Here's how the part is built. I have some questions about the finished solid (model axes, mm). Round coordinates to 2 decimals unless told otherwise and drop trailing zeros. Order: outer loops, then holes, each group sorted by start corner. A loop starts at its lowest first (then second) coordinate and runs counter-clockwise, first axis right, second up. Notation, with made-up numbers: (33, 86.5) -> (69, 86.5) arc R19 cw to (69, 94.5) -> close; hole circle Ø3 at (-19, -23.75). An arc over 180 degrees is marked (long way). Use a Markdown table: item, result. Add a question column.
(1) I want a section at A-A, the plane y = 4. Please give me the cut outline in (x, z), then the cut area to 3 significant figures.
(2) If I drill on probe 1 along Z at (x, y) = (-24.5, 3.75); probe 2 along Z at (x, y) = (9.5, 6); probe 3 along Y at (x, z) = (-14.5, 34.5), over which ranges is the centre line in solid material (lowest first)?
(3) I want a section at B-B, the plane x = 15. Please give me the cut outline in (y, z), then the cut area to 3 significant figures.
(4) I'm going to push a flat-ended pin straight in: P1, Ø2, axis at x = 0.5, z = 37.5, coming from the +Y side. Where does the tip first touch, or does it pass through?
from build123d import *

# Parameters (mm, degrees)
SKETCH1_W           = 80.5
SKETCH1_H           = 80
BOSS_EXTRUDE1_DEPTH = 10
CUT_EXTRUDE1_START  = -10
SKETCH2_W           = 11
SKETCH2_H           = 5
CUT_EXTRUDE1_DEPTH  = 60
CUT_EXTRUDE2_START  = -10
SKETCH3_W           = 2
SKETCH3_H           = 2
CUT_EXTRUDE2_DEPTH  = 60


with BuildPart() as part:
    # Sketch1 → Boss-Extrude1 (new body)
    with BuildSketch(Plane(origin=(0, 0, 0), x_dir=(1, 0, 0), z_dir=(0, 1, 0))):
        Rectangle(SKETCH1_W, SKETCH1_H)
    extrude(amount=BOSS_EXTRUDE1_DEPTH)

    # Sketch2 → Cut-Extrude1 (cut)
    with BuildSketch(Plane.ZY.offset(40.25).offset(CUT_EXTRUDE1_START)):
        with Locations((34.5, 7.5)):
            Rectangle(SKETCH2_W, SKETCH2_H)
    extrude(amount=-CUT_EXTRUDE1_DEPTH, mode=Mode.SUBTRACT)

    # Sketch3 → Cut-Extrude2 (cut)
    with BuildSketch(Plane.ZY.offset(40.25).offset(CUT_EXTRUDE2_START)):
        with Locations((37, 4)):
            Rectangle(SKETCH3_W, SKETCH3_H)
    extrude(amount=-CUT_EXTRUDE2_DEPTH, mode=Mode.SUBTRACT)


solid = part.part
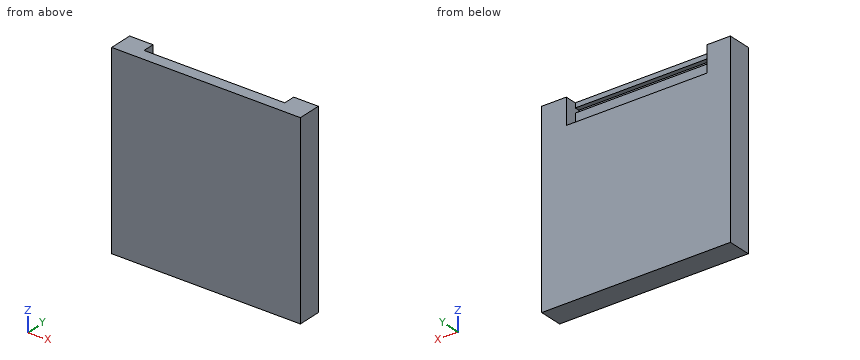
Taken from the geometry:
| question | item | result |
|---|---|---|
| 1 | outline | (-40.25, -40) -> (40.25, -40) -> (40.25, 40) -> (-40.25, 40) -> close; hole (-30.25, 36) -> (29.75, 36) -> (29.75, 38) -> (-30.25, 38) -> close |
| 1 | area | 6,320 mm2 |
| 2 | probe 1 | z = -40 to 36, 38 to 40 |
| 2 | probe 2 | z = -40 to 29 |
| 2 | probe 3 | y = 0 to 5 |
| 3 | outline | (0, -40) -> (10, -40) -> (10, 29) -> (5, 29) -> (5, 36) -> (3, 36) -> (3, 38) -> (5, 38) -> (5, 40) -> (0, 40) -> close |
| 3 | area | 741 mm2 |
| 4 | P1 | stops at y = 5 |
